Autodesk Inventor part; units mm, degrees
ref_plane "Work Plane1" through (-66, 0, -50) normal (0, 0, 1) x (1, 0, 0)
ref_plane "YZ Plane" through (0, 0, 0) normal (1, 0, 0) x (0, 1, 0)
ref_plane "XZ Plane" through (0, 0, 0) normal (0, 1, 0) x (-1, 0, 0)
sketch "Sketch1" plane through (0, 0, 0) normal (0, 1, 0) x (-1, 0, 0)
  line L0 (0, 0) -> (0, -100)
  line L1 (0, -100) -> (66, -100)
  line L2 (66, -100) -> (66, -70)
  line L3 (66, -70) -> (94, -70)
  line L4 (94, -70) -> (94, -30)
  line L5 (94, -30) -> (66, -30)
  line L6 (66, -30) -> (66, 0)
  line L7 (66, 0) -> (0, 0)
  dimension "d0" = 100
  dimension "d2" = 30
  dimension "d4" = 40
  dimension "d7" = 66
  dimension "d27" = 94
extrude "Extrusion1" add sketch "Sketch1" along normal blind 2
ref_plane "Work Plane1" through (-66, 0, -50) normal (0, 0, 1) x (1, 0, 0)
sketch "Sketch2" plane through (0, 0, 0) normal (0, -1, 0) x (1, 0, 0)
  point P0 (0, 0)
  point P1 (-69.9994, -37.5)
  point P2 (-90, -37.5)
  point P3 (-69.9994, -62.5)
  point P4 (-90, -62.5)
hole "Hole1" at (-90, 0, -37.5) at (-69.9994, 0, -37.5) at (-69.9994, 0, -62.5) at (-90, 0, -62.5) direction (0, 1, 0) diameter 3.1 end through all
chamfer "Chamfer1" distance 1.5 angle 45 4 edges at (-90, 0, -60.95) (-69.9994, 0, -60.95) (-69.9994, 0, -35.95) (-90, 0, -35.95) measured on face at (-22.8202, 0, -45.8956)
chamfer "Chamfer2" distance 2 angle 45 1 edges at (-94, 0, -50)
sketch "Sketch3" plane through (-66, 0, -50) normal (0, 0, 1) x (1, 0, 0)
  line L0 (66, -6) -> (58, -6)
  line L1 (58, -6) -> (45.307, 15.985)
  line L2 (66, 0) -> (66, 2)
  line L3 (0, 0) -> (66, 0)
  line L4 (45.307, 15.985) -> (66, 15.985)
  line L5 (66, 15.985) -> (66, -6)
  line L6 (66, -6) -> (66, -6)
  point P0 (66, 1)
  dimension "d22" = 8
  dimension "d23" = 120
  dimension "d24" = 6
extrude "Extrusion2" cut sketch "Sketch3" along normal through all both and the other way through all
chamfer "Chamfer3" distance 1 distance2 1.2 2 edges at (-66, 2, -15) (-66, 2, -85) measured on face at (-31.2626, 2, -46.0165)
sketch "Sketch4" plane through (0, 0, 0) normal (0, -1, 0) x (1, 0, 0)
  line L0 (-67.7565, -100) -> (-11.4641, -100)
  line L1 (-11.4641, -100) -> (-11.4641, 0)
  line L2 (-11.4641, 0) -> (-67.7565, 0)
  point P0 (0, 0)
  point P1 (-53.4039, -92)
  point P2 (-53.4039, -8)
  point P3 (-11.4641, 0)
  dimension "d31" = 8
  dimension "d32" = 41.9398
  dimension "d33" = 41.9398
  dimension "d34" = 8
  dimension "d35" = 100
hole "Hole2" at (-53.4039, 0, -92) at (-53.4039, 0, -8) direction (0, 1, 0) diameter 3.1 end through all
chamfer "Chamfer4" distance 1.5 angle 45 2 edges at (-53.4039, 0, -90.45) (-53.4039, 0, -6.45) measured on face at (-29.9666, 0, -45.9559)
sketch "Sketch6" plane through (0, 2, 0) normal (0, 1, 0) x (1, 0, 0)
  line L0 (-11.4641, 100) -> (-11.4641, 0)
  line L1 (-12.6188, 100) -> (-11.4641, 100)
  line L2 (-12.6188, 0) -> (-12.6188, 100)
  line L3 (-11.4641, 0) -> (-12.6188, 0)
  line L4 (-12.6188, 100) -> (-65, 100)
  line L5 (-65, 0) -> (-12.6188, 0)
  line L6 (-12.6715, 100) -> (-66, 100)
  line L7 (-11.4641, 100) -> (-11.4641, 39.7608)
  point P0 (-25.8771, 42.265)
  point P1 (-25.8771, 65.3)
  point P2 (-33.7057, 88)
  point P3 (-26.8923, 12)
  dimension "d56" = 34.7
  dimension "d57" = 42.265
  dimension "d83" = 21.0869
  dimension "d84" = 12
  dimension "d85" = 12
  dimension "d87" = 14.2735
  dimension "d88" = 14.413
  dimension "d89" = 14.413
hole "Hole3" at (-33.7057, 2, -88) at (-25.8771, 2, -65.3) at (-25.8771, 2, -42.265) at (-26.8923, 2, -12) direction (0, -1, 0) diameter 3.1 end through all
sketch "Sketch7" plane through (0, 0, 0) normal (0, -1, 0) x (1, 0, 0)
  point P0 (0, 0)
sketch "Sketch8" plane through (0, 0, 0) normal (0, -1, 0) x (1, 0, 0)
  point P0 (0, 0)
  point P1 (-17.8084, -91.4246)
  point P2 (-17.8084, -9.1996)
  point P3 (-89, -50)
  point P4 (-17.8084, -9.1996)
  point P5 (-17.8084, -91.4246)
  point P6 (-89, -50)
hole "Hole4" at (-17.8084, 0, -9.1996) at (-17.8084, 0, -91.4246) at (-89, 0, -50) direction (0, 1, 0) diameter 6 end through all
sketch "Sketch10" plane through (0, 2, 0) normal (0, 1, 0) x (1, 0, 0)
  line L0 (-65, 0) -> (-12.6188, 0)
  line L1 (-11.4641, 100) -> (-11.4641, 0)
  point P0 (0, 0)
  point P1 (-57.9417, 16.5491)
  point P2 (-57.9417, 16.5491)
  point P3 (-45.6452, 89.3147)
  point P4 (-21.1671, 27.553)
  dimension "d91" = 9.703
  dimension "d92" = 27.553
hole "Hole6" at (-21.1671, 2, -27.553) at (-45.6452, 2, -89.3147) at (-57.9417, 2, -16.5491) direction (0, -1, 0) diameter 3.1 end through all
properties part number "podstawa" material "Steel"
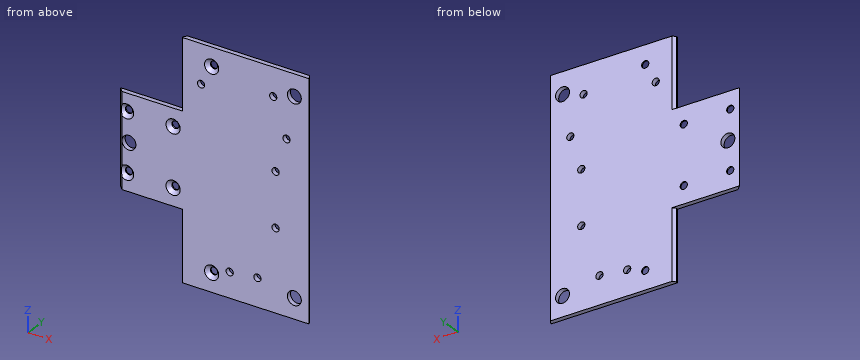
Verification items for the finished model (mm, model axes). Give positions to 0.01 mm unless a question says otherwise; leave off trailing zeros. Order: outer loops, then holes, each group sorted by start corner. A loop starts at its lowest first (then second) coordinate and runs counter-clockwise, first axis right, second up. Notation, with made-up numbers: M 47.25,86.25 L 98.25,86.25 A25 cw 98.25,116.25 Z; hole C 39,33 d7. An arc over 180 degrees is marked long. Use one line per item in the form item = value. Start each with the question number.
Q1. Section check A-A (z = -92). Enter the section's corners in (x, y), then the cut area to 3 significant figures.
Q2. Section check B-B (z = -68.5). Enter the section's corners in (x, y), then the cut area to 3 significant figures.
Q3. Scan lines: line 1 along Z through (x, y) = (-90, 1.85); line 2 along Z through (x, y) = (-54, 1.3); line 3 along Z through (x, y) = (-53, 0.55). Record each from-to range of solid material in increasing order. Write a range as [from, to].
Q4. Section check C-C (z = -37.5). Enter the section's corners in (x, y) (3 decimals), then the cut area to 3 significant figures.
Q5. Go/stop test with flat-tipped pins: pin 1 Ø5 at (x, z) = (-25.88, -42.26) entering from +Y; pin 2 Ø2.5 at (x, z) = (-70, -62.5) entering from -Y; pin 3 Ø0.9 at (y, z) = (0.5, -17) entering from -X; pin 4 Ø1 at (x, y) = (-77.5, 1) entering from +Z. Record where each tip stops, or that it passes through.
Evaluation:
q1.outline = M -66,0 L -56.45,0 L -54.95,1.5 L -54.95,2 L -65,2 L -66,0.8 Z; M -51.85,1.5 L -50.35,0 L -20.75,0 L -20.75,2 L -51.85,2 Z; M -14.86,0 L -11.46,0 L -12.62,2 L -14.86,2 Z
q1.area = 87.1 mm2
q2.outline = M -94,2 L -92,0 L -11.46,0 L -12.62,2 Z
q2.area = 162 mm2
q3.line_1 = [-70, -64.05], [-60.95, -52.83], [-47.17, -39.05], [-35.95, -30]
q3.line_2 = [-100, -93.65], [-90.35, -9.65], [-6.35, 0]
q3.line_3 = [-100, -94.47], [-89.53, -10.47], [-5.53, 0]
q4.outline = M -94,2 L -92.525,0.525 L -91.55,1.5 L -91.55,2 Z; M -88.45,1.5 L -86.95,0 L -73.049,0 L -71.549,1.5 L -71.549,2 L -88.45,2 Z; M -68.449,1.5 L -66.949,0 L -11.464,0 L -12.619,2 L -68.449,2 Z
q4.area = 145 mm2
q5.pin_1 = 2
q5.pin_2 = through
q5.pin_3 = -66
q5.pin_4 = -30
